```python
from build123d import *

# Parameters (mm, degrees)
SKETCH2_W                      = 78.0542
SKETCH2_H                      = 84.0867
SKETCH2_W_2                    = 70.3326
SKETCH2_H_2                    = 75.8698
BOSS_EXTRUDE1_DEPTH            = 24.0665
F_7_16_0_4375_DIAMETER_HOLE1_D = 11.1125
F_7_16_0_4375_DIAMETER_HOLE2_D = 11.1125
FILLET2_R                      = 6.35
FILLET3_R                      = 2.54
F_4_40_TAPPED_HOLE1_D          = 2.2606
F_4_40_TAPPED_HOLE1_DEPTH      = 3.8608
F_4_40_TAPPED_HOLE2_D          = 2.2606


with BuildPart() as part:
    # Sketch2 → Boss-Extrude1 (new body)
    with BuildSketch(Plane.XY):
        Rectangle(SKETCH2_W, SKETCH2_H)
        Rectangle(SKETCH2_W_2, SKETCH2_H_2, mode=Mode.SUBTRACT)
    extrude(amount=BOSS_EXTRUDE1_DEPTH)

    # 7/16 (0.4375) Diameter Hole1 (through all)
    with Locations(Plane.ZY.offset(39.0271)):
        with Locations((12.03325, 0)):
            Hole(F_7_16_0_4375_DIAMETER_HOLE1_D / 2)

    # 7/16 (0.4375) Diameter Hole2 (through all)
    with Locations(Plane(origin=(0, 42.04335, 0), x_dir=(1, 0, 0), z_dir=(0, 1, 0))):
        with Locations((0, -12.03325)):
            Hole(F_7_16_0_4375_DIAMETER_HOLE2_D / 2)

    # Fillet2
    fillet2_edges = [part.edges().sort_by_distance(p)[0] for p in [
        (39.0271, -42.04335, 12.03325),
        (-39.0271, -42.04335, 12.03325),
        (-39.0271, 42.04335, 12.03325),
        (39.0271, 42.04335, 12.03325),
    ]]
    fillet(fillet2_edges, radius=FILLET2_R)

    # Fillet3
    fillet3_edges = [part.edges().sort_by_distance(p)[0] for p in [
        (35.1663, -37.9349, 12.03325),
        (35.1663, 37.9349, 12.03325),
        (-35.1663, 37.9349, 12.03325),
        (-35.1663, -37.9349, 12.03325),
    ]]
    fillet(fillet3_edges, radius=FILLET3_R)

    # #4-40 Tapped Hole1
    with Locations(Plane(origin=(39.0271, 0, 0), x_dir=(0, 0, -1), z_dir=(1, 0, 0))):
        with Locations((-12.03325, 23.241), (-12.03325, -23.241)):
            Hole(F_4_40_TAPPED_HOLE1_D / 2, depth=F_4_40_TAPPED_HOLE1_DEPTH)

    # #4-40 Tapped Hole2 (through all)
    with Locations(Plane(origin=(0, -42.04335, 0), x_dir=(-1, 0, 0), z_dir=(0, -1, 0))):
        with Locations((-30.1371, -12.03325), (30.1371, -12.03325)):
            Hole(F_4_40_TAPPED_HOLE2_D / 2)


solid = part.part
```
Input: part model. Units: mm. Frame: model coordinates. A direction names the side the tool comes from. Coordinates: 2 decimals unless noted, no trailing zeros. Order: outer loops, then holes, each group sorted by start corner. A loop starts at its lowest first (then second) coordinate and runs counter-clockwise, first axis right, second up. Notation, with made-up numbers: (-17.5, 25) - (32.5, 25) arc R25 ccw to (32.5, 48) - close; hole circle Ø7 at (87.5, 89). An arc over 180 degrees is marked (long way). Put each result on its own line as item: value.
1. Cut plane C-C on z = 4.25. Return the cut outline in (x, y).
Report:
outline: (-39.03, -35.69) arc R6.35 ccw to (-32.68, -42.04) - (32.68, -42.04) arc R6.35 ccw to (39.03, -35.69) - (39.03, 35.69) arc R6.35 ccw to (32.68, 42.04) - (-32.68, 42.04) arc R6.35 ccw to (-39.03, 35.69) - close; hole (-35.17, -35.39) arc R2.54 ccw to (-32.63, -37.93) - (32.63, -37.93) arc R2.54 ccw to (35.17, -35.39) - (35.17, 35.39) arc R2.54 ccw to (32.63, 37.93) - (-32.63, 37.93) arc R2.54 ccw to (-35.17, 35.39) - close
2. Line query: line 1 along Y through (x, z) = (-5, 19.25); line 2 along X through (y, z) = (-10, 9.75); line 3 along Z through (x, y) = (0, -41.1). Output: solid intervals per line, ascending.
Report:
line 1: y = -42.04 to -37.93, 37.93 to 42.04
line 2: x = -39.03 to -35.17, 35.17 to 39.03
line 3: z = 0 to 6.48, 17.59 to 24.07
3. Cut plane A-A on y = -12. Return the cut outline in (x, z).
Report:
outline: (-39.03, 0) - (-35.17, 0) - (-35.17, 24.07) - (-39.03, 24.07) - close; (35.17, 0) - (39.03, 0) - (39.03, 24.07) - (35.17, 24.07) - close
4. Cut plane D-D on x = -25. Return the cut outline in (y, z), then the cut area to 3 significant figures.
Report:
outline: (-42.04, 0) - (-37.93, 0) - (-37.93, 24.07) - (-42.04, 24.07) - close; (37.93, 0) - (42.04, 0) - (42.04, 24.07) - (37.93, 24.07) - close
area: 198 mm2
5. Contact query for flat-ended pins moving along their axis: pin 1 Ø2 at (y, z) = (-23.24, 12.03) entering from +X; pin 2 Ø6.5 at (y, z) = (0, 12.03) entering from -X. Output: stop coordinate, or through.
Report:
pin 1: stops at x = -35.17
pin 2: passes through
6. Draft query along X for faces 1 (the face through (-37.07, 0.244, 17.584)), 2 (the face through (39.027, 7, 12)), 3 (the face through (7, -37.935, 12)). Return one class per face: pulls with the +X half, pulls with the -X half, needs draft (parallel to the pull), parting line crosses it, or undercut.
Report:
face 1: needs draft
face 2: pulls with the +X half
face 3: undercut
7. Cut plane B-B on x = 0. Return the cut outline in (y, z).
Report:
outline: (-42.04, 0) - (-37.93, 0) - (-37.93, 6.48) - (-42.04, 6.48) - close; (-42.04, 17.59) - (-37.93, 17.59) - (-37.93, 24.07) - (-42.04, 24.07) - close; (37.93, 0) - (42.04, 0) - (42.04, 6.48) - (37.93, 6.48) - close; (37.93, 17.59) - (42.04, 17.59) - (42.04, 24.07) - (37.93, 24.07) - close
8. Reachability of faces 4 (the face through (7, -42.043, 12)), 5 (the face through (-35.166, -8, 12)), 6 (the face through (37.07, 22.138, 11.788)) from +Z, -Z, +X, -X, +Y, -Y: full face, straight path, thin tool, end or side. Return the list, or none.
Report:
face 4: +Z, -Z, +X, -X, -Y
face 5: +Z, -Z
face 6: +X
